Geometry: final body of the model. Coordinates: model frame, mm. Face numbers are marked on the shaded views. Coordinates: 2 decimals unless noted, no trailing zeros. Loops run counter-clockwise (first coordinate to the right, second up) from the corner with the lowest first, then second, coordinate; pieces in that order, holes last. Notation, with made-up numbers: (1, 26) - (51, 26) arc R23 cw to (51, 54) - close; hole circle Ø4 at (50.25, 74). An arc over 180 degrees is marked (long way). Write each question's results on one line, items separated by ' | '. Start each with the question number.
from build123d import *

# Parameters (mm, degrees)
SKETCH1_W                 = 90.17
SKETCH1_H                 = 95.885
BOSS_EXTRUDE1_DEPTH       = 51
SKETCH2_R                 = 1.5875
CUT_EXTRUDE1_DEPTH        = 51
SKETCH3_R                 = 13.25
CUT_EXTRUDE2_DEPTH        = 51
LPATTERN1_COUNT           = 3
LPATTERN1_PITCH           = 29
LPATTERN2_COUNT           = 3
LPATTERN2_PITCH           = 28
LPATTERN2_COPY_1_SKETCH_R = 13.25
LPATTERN2_COPY_1_DEPTH    = 51
LPATTERN2_COPY_2_SKETCH_R = 13.25
LPATTERN2_COPY_2_DEPTH    = 51
LPATTERN2_COPY_3_SKETCH_R = 13.25
LPATTERN2_COPY_3_DEPTH    = 51
LPATTERN2_COPY_4_SKETCH_R = 13.25
LPATTERN2_COPY_4_DEPTH    = 51
SKETCH4_W                 = 1.872435897
SKETCH4_H                 = 0.651282051
BOSS_EXTRUDE2_DEPTH       = 0.01
SKETCH6_W                 = 5
SKETCH6_H                 = 10
CUT_EXTRUDE3_DEPTH        = 3
LPATTERN3_COUNT           = 2
LPATTERN3_PITCH           = 29
LPATTERN4_COUNT           = 3
LPATTERN4_PITCH           = 28
LPATTERN4_COPY_1_SKETCH_W = 5
LPATTERN4_COPY_1_SKETCH_H = 10
LPATTERN4_COPY_1_DEPTH    = 3
LPATTERN4_COPY_2_SKETCH_W = 5
LPATTERN4_COPY_2_SKETCH_H = 10
LPATTERN4_COPY_2_DEPTH    = 3
SKETCH7_W                 = 8.328938764
SKETCH7_H                 = 5
CUT_EXTRUDE4_DEPTH        = 3
LPATTERN5_COUNT           = 2
LPATTERN5_PITCH           = 28
LPATTERN6_COUNT           = 3
LPATTERN6_PITCH           = 29
LPATTERN6_COPY_1_SKETCH_W = 8.328938764
LPATTERN6_COPY_1_SKETCH_H = 5
LPATTERN6_COPY_1_DEPTH    = 3
LPATTERN6_COPY_2_SKETCH_W = 8.328938764
LPATTERN6_COPY_2_SKETCH_H = 5
LPATTERN6_COPY_2_DEPTH    = 3
MIRROR2_COPY_1_SKETCH_W   = 5
MIRROR2_COPY_1_SKETCH_H   = 10
MIRROR2_COPY_1_DEPTH      = 3
MIRROR2_COPY_2_SKETCH_W   = 5
MIRROR2_COPY_2_SKETCH_H   = 10
MIRROR2_COPY_2_DEPTH      = 3
MIRROR2_COPY_3_SKETCH_W   = 5
MIRROR2_COPY_3_SKETCH_H   = 10
MIRROR2_COPY_3_DEPTH      = 3
MIRROR2_COPY_4_SKETCH_W   = 5
MIRROR2_COPY_4_SKETCH_H   = 10
MIRROR2_COPY_4_DEPTH      = 3
MIRROR2_COPY_5_SKETCH_W   = 5
MIRROR2_COPY_5_SKETCH_H   = 10
MIRROR2_COPY_5_DEPTH      = 3
MIRROR2_COPY_6_SKETCH_W   = 8.328938764
MIRROR2_COPY_6_SKETCH_H   = 5
MIRROR2_COPY_6_DEPTH      = 3
MIRROR2_COPY_7_SKETCH_W   = 8.328938764
MIRROR2_COPY_7_SKETCH_H   = 5
MIRROR2_COPY_7_DEPTH      = 3
MIRROR2_COPY_8_SKETCH_W   = 8.328938764
MIRROR2_COPY_8_SKETCH_H   = 5
MIRROR2_COPY_8_DEPTH      = 3
MIRROR2_COPY_9_SKETCH_W   = 8.328938764
MIRROR2_COPY_9_SKETCH_H   = 5
MIRROR2_COPY_9_DEPTH      = 3
MIRROR2_COPY_10_SKETCH_W  = 8.328938764
MIRROR2_COPY_10_SKETCH_H  = 5
MIRROR2_COPY_10_DEPTH     = 3


with BuildPart() as part:
    # Sketch1 → Boss-Extrude1 (new body)
    with BuildSketch(Plane(origin=(0, 0, 0), x_dir=(1, 0, 0), z_dir=(0, 1, 0))):
        Rectangle(SKETCH1_W, SKETCH1_H)
    extrude(amount=BOSS_EXTRUDE1_DEPTH)

    # Sketch2 → Cut-Extrude1 (cut)
    with BuildSketch(Plane(origin=(0, 51, 0), x_dir=(1, 0, 0), z_dir=(0, 1, 0))):
        with Locations(Location((-36.195, 42.8625, 0), (0, 0, 270))):
            Circle(SKETCH2_R)
        with Locations(Location((37.465, 42.8625, 0), (0, 0, 270))):
            Circle(SKETCH2_R)
        with Locations(Location((-40.005, -42.8625, 0), (0, 0, 270))):
            Circle(SKETCH2_R)
        with Locations(Location((40.005, -42.8625, 0), (0, 0, 270))):
            Circle(SKETCH2_R)
    extrude(amount=-CUT_EXTRUDE1_DEPTH, mode=Mode.SUBTRACT)

    # Sketch3 → Cut-Extrude2 (cut)
    with BuildSketch(Plane(origin=(0, 51, 0), x_dir=(1, 0, 0), z_dir=(0, 1, 0))):
        with Locations(Location((-27.085, -29.9425, 0), (0, 0, 270))):
            Circle(SKETCH3_R)
    cut_extrude2 = extrude(amount=-CUT_EXTRUDE2_DEPTH, mode=Mode.SUBTRACT)

    # LPattern1: Cut-Extrude2 ×3
    with Locations(*[(0, 0, -i * LPATTERN1_PITCH) for i in range(1, LPATTERN1_COUNT)]):
        add(cut_extrude2, mode=Mode.SUBTRACT)

    # LPattern2: Cut-Extrude2 ×3
    with Locations(*[(i * LPATTERN2_PITCH, 0, 0) for i in range(1, LPATTERN2_COUNT)]):
        add(cut_extrude2, mode=Mode.SUBTRACT)

    # LPattern2 copy 1 sketch → LPattern2 copy 1 (cut)
    with BuildSketch(Plane(origin=(28, 51, -29), x_dir=(1, 0, 0), z_dir=(0, 1, 0))):
        with Locations(Location((-27.085, -29.9425, 0), (0, 0, 270))):
            Circle(LPATTERN2_COPY_1_SKETCH_R)
    extrude(amount=-LPATTERN2_COPY_1_DEPTH, mode=Mode.SUBTRACT)

    # LPattern2 copy 2 sketch → LPattern2 copy 2 (cut)
    with BuildSketch(Plane(origin=(56, 51, -29), x_dir=(1, 0, 0), z_dir=(0, 1, 0))):
        with Locations(Location((-27.085, -29.9425, 0), (0, 0, 270))):
            Circle(LPATTERN2_COPY_2_SKETCH_R)
    extrude(amount=-LPATTERN2_COPY_2_DEPTH, mode=Mode.SUBTRACT)

    # LPattern2 copy 3 sketch → LPattern2 copy 3 (cut)
    with BuildSketch(Plane(origin=(28, 51, -58), x_dir=(1, 0, 0), z_dir=(0, 1, 0))):
        with Locations(Location((-27.085, -29.9425, 0), (0, 0, 270))):
            Circle(LPATTERN2_COPY_3_SKETCH_R)
    extrude(amount=-LPATTERN2_COPY_3_DEPTH, mode=Mode.SUBTRACT)

    # LPattern2 copy 4 sketch → LPattern2 copy 4 (cut)
    with BuildSketch(Plane(origin=(56, 51, -58), x_dir=(1, 0, 0), z_dir=(0, 1, 0))):
        with Locations(Location((-27.085, -29.9425, 0), (0, 0, 270))):
            Circle(LPATTERN2_COPY_4_SKETCH_R)
    extrude(amount=-LPATTERN2_COPY_4_DEPTH, mode=Mode.SUBTRACT)

    # Sketch4 → Boss-Extrude2 (add)
    with BuildSketch(Plane.XY.offset(47.9425)):
        Polygon((-40.935431089, 46.473214492), (-40.359199118, 46.473214492), (-39.144405448, 43.85663797), (-37.929611778, 46.473214492), (-37.353379807, 46.473214492), (-38.900174678, 43.141754156), (-38.900174678, 40.123214492), (-39.388636217, 40.123214492), (-39.388636217, 43.141754156), align=None)
        with Locations((-36.172931089, 42.565522184)):
            Rectangle(SKETCH4_W, SKETCH4_H)
    extrude(amount=BOSS_EXTRUDE2_DEPTH)

    # Sketch6 → Cut-Extrude3 (cut)
    with BuildSketch(Plane(origin=(0, 51, 0), x_dir=(1, 0, 0), z_dir=(0, 1, 0))):
        with Locations((-27.085, -15.4425)):
            Rectangle(SKETCH6_W, SKETCH6_H)
    cut_extrude3 = extrude(amount=-CUT_EXTRUDE3_DEPTH, mode=Mode.SUBTRACT)

    # LPattern3: Cut-Extrude3 ×2
    with Locations(*[(0, 0, -i * LPATTERN3_PITCH) for i in range(1, LPATTERN3_COUNT)]):
        add(cut_extrude3, mode=Mode.SUBTRACT)

    # LPattern4: Cut-Extrude3 ×3
    with Locations(*[(i * LPATTERN4_PITCH, 0, 0) for i in range(1, LPATTERN4_COUNT)]):
        add(cut_extrude3, mode=Mode.SUBTRACT)

    # LPattern4 copy 1 sketch → LPattern4 copy 1 (cut)
    with BuildSketch(Plane(origin=(28, 51, -29), x_dir=(1, 0, 0), z_dir=(0, 1, 0))):
        with Locations((-27.085, -15.4425)):
            Rectangle(LPATTERN4_COPY_1_SKETCH_W, LPATTERN4_COPY_1_SKETCH_H)
    extrude(amount=-LPATTERN4_COPY_1_DEPTH, mode=Mode.SUBTRACT)

    # LPattern4 copy 2 sketch → LPattern4 copy 2 (cut)
    with BuildSketch(Plane(origin=(56, 51, -29), x_dir=(1, 0, 0), z_dir=(0, 1, 0))):
        with Locations((-27.085, -15.4425)):
            Rectangle(LPATTERN4_COPY_2_SKETCH_W, LPATTERN4_COPY_2_SKETCH_H)
    extrude(amount=-LPATTERN4_COPY_2_DEPTH, mode=Mode.SUBTRACT)

    # Sketch7 → Cut-Extrude4 (cut)
    with BuildSketch(Plane(origin=(0, 51, 0), x_dir=(1, 0, 0), z_dir=(0, 1, 0))):
        with Locations((-13.085, -29.9425)):
            Rectangle(SKETCH7_W, SKETCH7_H)
    cut_extrude4 = extrude(amount=-CUT_EXTRUDE4_DEPTH, mode=Mode.SUBTRACT)

    # LPattern5: Cut-Extrude4 ×2
    with Locations(*[(i * LPATTERN5_PITCH, 0, 0) for i in range(1, LPATTERN5_COUNT)]):
        add(cut_extrude4, mode=Mode.SUBTRACT)

    # LPattern6: Cut-Extrude4 ×3
    with Locations(*[(0, 0, -i * LPATTERN6_PITCH) for i in range(1, LPATTERN6_COUNT)]):
        add(cut_extrude4, mode=Mode.SUBTRACT)

    # LPattern6 copy 1 sketch → LPattern6 copy 1 (cut)
    with BuildSketch(Plane(origin=(28, 51, -29), x_dir=(1, 0, 0), z_dir=(0, 1, 0))):
        with Locations((-13.085, -29.9425)):
            Rectangle(LPATTERN6_COPY_1_SKETCH_W, LPATTERN6_COPY_1_SKETCH_H)
    extrude(amount=-LPATTERN6_COPY_1_DEPTH, mode=Mode.SUBTRACT)

    # LPattern6 copy 2 sketch → LPattern6 copy 2 (cut)
    with BuildSketch(Plane(origin=(28, 51, -58), x_dir=(1, 0, 0), z_dir=(0, 1, 0))):
        with Locations((-13.085, -29.9425)):
            Rectangle(LPATTERN6_COPY_2_SKETCH_W, LPATTERN6_COPY_2_SKETCH_H)
    extrude(amount=-LPATTERN6_COPY_2_DEPTH, mode=Mode.SUBTRACT)

    # Mirror2: Cut-Extrude3, Cut-Extrude4 across plane
    add(cut_extrude3.mirror(Plane.ZX.offset(25.5)), mode=Mode.SUBTRACT)
    add(cut_extrude4.mirror(Plane.ZX.offset(25.5)), mode=Mode.SUBTRACT)

    # Mirror2 copy 1 sketch → Mirror2 copy 1 (cut)
    with BuildSketch(Plane(origin=(0, 0, -29), x_dir=(1, 0, 0), z_dir=(0, -1, 0))):
        with Locations((-27.085, 15.4425)):
            Rectangle(MIRROR2_COPY_1_SKETCH_W, MIRROR2_COPY_1_SKETCH_H)
    extrude(amount=-MIRROR2_COPY_1_DEPTH, mode=Mode.SUBTRACT)

    # Mirror2 copy 2 sketch → Mirror2 copy 2 (cut)
    with BuildSketch(Plane(origin=(28, 0, 0), x_dir=(1, 0, 0), z_dir=(0, -1, 0))):
        with Locations((-27.085, 15.4425)):
            Rectangle(MIRROR2_COPY_2_SKETCH_W, MIRROR2_COPY_2_SKETCH_H)
    extrude(amount=-MIRROR2_COPY_2_DEPTH, mode=Mode.SUBTRACT)

    # Mirror2 copy 3 sketch → Mirror2 copy 3 (cut)
    with BuildSketch(Plane(origin=(56, 0, 0), x_dir=(1, 0, 0), z_dir=(0, -1, 0))):
        with Locations((-27.085, 15.4425)):
            Rectangle(MIRROR2_COPY_3_SKETCH_W, MIRROR2_COPY_3_SKETCH_H)
    extrude(amount=-MIRROR2_COPY_3_DEPTH, mode=Mode.SUBTRACT)

    # Mirror2 copy 4 sketch → Mirror2 copy 4 (cut)
    with BuildSketch(Plane(origin=(28, 0, -29), x_dir=(1, 0, 0), z_dir=(0, -1, 0))):
        with Locations((-27.085, 15.4425)):
            Rectangle(MIRROR2_COPY_4_SKETCH_W, MIRROR2_COPY_4_SKETCH_H)
    extrude(amount=-MIRROR2_COPY_4_DEPTH, mode=Mode.SUBTRACT)

    # Mirror2 copy 5 sketch → Mirror2 copy 5 (cut)
    with BuildSketch(Plane(origin=(56, 0, -29), x_dir=(1, 0, 0), z_dir=(0, -1, 0))):
        with Locations((-27.085, 15.4425)):
            Rectangle(MIRROR2_COPY_5_SKETCH_W, MIRROR2_COPY_5_SKETCH_H)
    extrude(amount=-MIRROR2_COPY_5_DEPTH, mode=Mode.SUBTRACT)

    # Mirror2 copy 6 sketch → Mirror2 copy 6 (cut)
    with BuildSketch(Plane(origin=(28, 0, 0), x_dir=(1, 0, 0), z_dir=(0, -1, 0))):
        with Locations((-13.085, 29.9425)):
            Rectangle(MIRROR2_COPY_6_SKETCH_W, MIRROR2_COPY_6_SKETCH_H)
    extrude(amount=-MIRROR2_COPY_6_DEPTH, mode=Mode.SUBTRACT)

    # Mirror2 copy 7 sketch → Mirror2 copy 7 (cut)
    with BuildSketch(Plane(origin=(0, 0, -29), x_dir=(1, 0, 0), z_dir=(0, -1, 0))):
        with Locations((-13.085, 29.9425)):
            Rectangle(MIRROR2_COPY_7_SKETCH_W, MIRROR2_COPY_7_SKETCH_H)
    extrude(amount=-MIRROR2_COPY_7_DEPTH, mode=Mode.SUBTRACT)

    # Mirror2 copy 8 sketch → Mirror2 copy 8 (cut)
    with BuildSketch(Plane(origin=(0, 0, -58), x_dir=(1, 0, 0), z_dir=(0, -1, 0))):
        with Locations((-13.085, 29.9425)):
            Rectangle(MIRROR2_COPY_8_SKETCH_W, MIRROR2_COPY_8_SKETCH_H)
    extrude(amount=-MIRROR2_COPY_8_DEPTH, mode=Mode.SUBTRACT)

    # Mirror2 copy 9 sketch → Mirror2 copy 9 (cut)
    with BuildSketch(Plane(origin=(28, 0, -29), x_dir=(1, 0, 0), z_dir=(0, -1, 0))):
        with Locations((-13.085, 29.9425)):
            Rectangle(MIRROR2_COPY_9_SKETCH_W, MIRROR2_COPY_9_SKETCH_H)
    extrude(amount=-MIRROR2_COPY_9_DEPTH, mode=Mode.SUBTRACT)

    # Mirror2 copy 10 sketch → Mirror2 copy 10 (cut)
    with BuildSketch(Plane(origin=(28, 0, -58), x_dir=(1, 0, 0), z_dir=(0, -1, 0))):
        with Locations((-13.085, 29.9425)):
            Rectangle(MIRROR2_COPY_10_SKETCH_W, MIRROR2_COPY_10_SKETCH_H)
    extrude(amount=-MIRROR2_COPY_10_DEPTH, mode=Mode.SUBTRACT)


solid = part.part
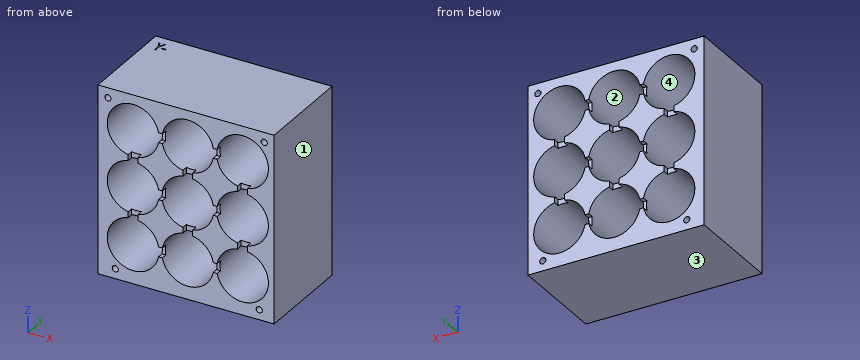
1) Pin query (flat end, axial travel): pin 1 Ø2 at (x, y) = (15.5, 49.5) entering from +Z; pin 2 Ø2.5 at (x, z) = (-27.5, 16) entering from +Y. Return the tip coordinate at first contact, or that it passes through.
2) Section query B-B on z = -5. Output: boundary loops of the cut face in (x, y) (3 decimals).
3) Section query A-A on x = 22. Output: boundary loops of the cut face in (y, z), and give its area (3 significant figures).
4) Section query C-C on y = 11.5. Count the separate pieces of the cut face and the enclosed holes in it, and give its area (3 significant figures).
5) Material intervals for line 1 (Z direction, x = 28.5, y = 31.5); line 2 (Z direction, x = 32, y = 34); line 3 (X direction, y = 38, z = 0) (3 decimals), sorted ascending. Write a range as [from, to].
6) Pull-direction query (X, two-part tool) for the marked faces 1, 2, 3 and 4; classes: released by +X, released by -X, zero draft, split by the parting line, or undercut.
Returned:
1) pin 1: stops at z = 47.94 | pin 2: stops at y = 48
2) outline: (-45.085, 0) - (-38.928, 0) - (-38.928, 51) - (-45.085, 51) - close; (-15.242, 0) - (-10.928, 0) - (-10.928, 51) - (-15.242, 51) - close; (12.758, 0) - (17.072, 0) - (17.072, 51) - (12.758, 51) - close; (40.758, 0) - (45.085, 0) - (45.085, 51) - (40.758, 51) - close
3) outline: (0, -47.94) - (51, -47.94) - (51, -39.36) - (0, -39.36) - close; (0, -16.76) - (51, -16.76) - (51, -10.36) - (0, -10.36) - close; (0, 12.24) - (51, 12.24) - (51, 18.64) - (0, 18.64) - close; (0, 41.24) - (51, 41.24) - (51, 47.94) - (0, 47.94) - close | area: 1,430 mm²
4) separate pieces: 1 | enclosed holes: 13 | area: 3,650 mm²
5) line 1: z = [-47.94, -41.3], [-14.81, -12.3], [14.19, 16.7], [43.19, 47.94] | line 2: z = [-47.94, -40.94], [-15.17, -11.94], [13.83, 17.06], [42.83, 47.94] | line 3: x = [-45.085, -40.301], [-13.869, -12.301], [14.131, 15.699], [42.131, 45.085]
6) face 1: released by +X | face 2: undercut | face 3: zero draft | face 4: undercut
